Source: three-view drawing plus pictorial views. Frame: mm from the lowest corner of the part. A direction names the side the tool comes from. Round coordinates to 2 decimals unless told otherwise and drop trailing zeros. Write each loop counter-clockwise with the first axis right and the second up, starting at its lowest first coordinate (ties: lowest second). Pieces come first, ordered by that corner, then holes. Notation, with made-up numbers: (-2, -28) -> (40, -28) arc R38 cw to (40, 10) -> close; hole circle Ø3 at (31, 18.25). An arc over 180 degrees is marked (long way). Put each result on its own line as item: value.
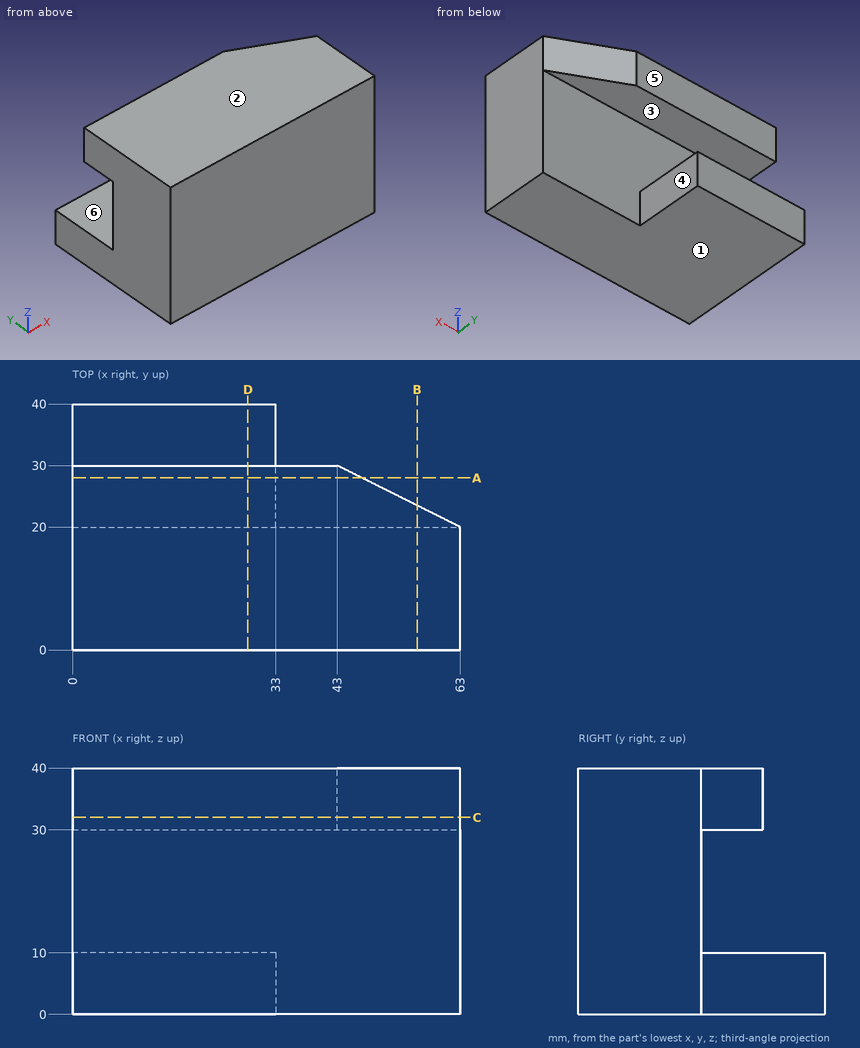
Q1. Cut plane B-B on x = 56. Output: boundary loops of the cut face in (y, z).
Ans:
outline: (0, 0) -> (20, 0) -> (20, 30) -> (23.5, 30) -> (23.5, 40) -> (0, 40) -> close
Q2. Cut plane D-D on x = 28.5. Output: boundary loops of the cut face in (y, z), and give its area (3 significant figures).
Ans:
outline: (0, 0) -> (40, 0) -> (40, 10) -> (20, 10) -> (20, 30) -> (30, 30) -> (30, 40) -> (0, 40) -> close
area: 1,100 mm^2
Q3. Material intervals for line 1 (Z direction, x = 25, y = 27); line 2 (Y direction, x = 28, z = 29); line 3 (Y direction, x = 14.5, z = 33.5), sorted ascending. Write a range as [from, to].
Ans:
line 1: z = [0, 10], [30, 40]
line 2: y = [0, 20]
line 3: y = [0, 30]
Q4. Cut plane C-C on z = 32. Output: boundary loops of the cut face in (x, y), and give its area (3 significant figures).
Ans:
outline: (0, 0) -> (63, 0) -> (63, 20) -> (43, 30) -> (0, 30) -> close
area: 1,790 mm^2
Q5. Cut plane A-A on y = 28. Output: boundary loops of the cut face in (x, z), and give its area (3 significant figures).
Ans:
outline: (0, 0) -> (33, 0) -> (33, 10) -> (0, 10) -> close; (0, 30) -> (47, 30) -> (47, 40) -> (0, 40) -> close
area: 800 mm^2
Q6. Pin query (flat end, axial travel): pin 1 (11 mm diameter, centred on y = 30, z = 4.5, fed in from +X); pin 2 (5 mm diameter, centred on y = 24.5, z = 31.5, fed in from +X); pin 3 (11 mm diameter, centred on x = 31, z = 34.5, fed in from +Y). Return the tip coordinate at first contact, or that it passes through.
Ans:
pin 1: stops at x = 33
pin 2: stops at x = 59
pin 3: stops at y = 30
Q7. Draft query along Z for the marked faces 1, 2 and 3. Return one class per face: +Z half, -Z half, draft (parallel to the pull), parting line (faces both ways), or undercut.
Ans:
face 1: -Z half
face 2: +Z half
face 3: undercut
Q8. Reachability of the marked faces 4, 5 and 6 from +Z, -Z, +X, -X, +Y, -Y: full face, straight path, thin tool, end or side. Return the list, or none.
Ans:
face 4: -Z, +X, +Y
face 5: +Z, +X, -X, +Y
face 6: +X, -X, +Y
